Geometry: final body of the model. Coordinates: model frame, mm. Face numbers are marked on the shaded views. A direction names the side the tool comes from. Coordinates: 2 decimals unless noted, no trailing zeros. Write each loop counter-clockwise with the first axis right and the second up, starting at its lowest first coordinate (ties: lowest second). Pieces come first, ordered by that corner, then holes. Notation, with made-up numbers: (19.5, 18.25) - (23.5, 18.25) arc R7 ccw to (23.5, 28.25) - close; hole circle Ø11 at (-20.75, 32). An arc over 180 degrees is marked (long way). Put each result on its own line as item: value.
```python
from build123d import *

# Parameters (mm, degrees)
F0_R     = 11.049
F1_DEPTH = 6.35


with BuildPart() as f1:
    # F0 (on Top) → F1 (new body)
    with BuildSketch(Plane.XY):
        with BuildLine():
            ThreePointArc((13.9900267073, 42.191013886), (7.0856169162, 43.8816195339), (1.001e-07, 44.45))
            ThreePointArc((1.001e-07, 44.45), (-8.1127014874, 43.7033931701), (-15.9528722093, 41.4886534883))
            ThreePointArc((-15.9528722093, 41.4886534883), (-18.8508822531, 32.2986856143), (-16.6280791163, 22.9224860668))
            ThreePointArc((-16.6280791163, 22.9224860668), (-15.8658789133, 20.1464210948), (-15.6090878752, 17.2790975622))
            ThreePointArc((-15.6090878752, 17.2790975622), (-17.5525161747, 9.6016065701), (-22.9146844129, 3.773405023))
            ThreePointArc((-22.9146844129, 3.773405023), (-24.5849396697, 2.8183178083), (-26.356998831, 2.0688176155))
            ThreePointArc((-26.356998831, 2.0688176155), (-36.5044925545, -0.529991355), (-43.6973944973, -8.1449502237))
            ThreePointArc((-43.6973944973, -8.1449502237), (-41.7877364398, -15.1521478094), (-38.7624793768, -21.7548314763))
            ThreePointArc((-38.7624793768, -21.7548314763), (-29.6282610574, -1.7859753114), (-12.3702381212, -15.3635231449))
            ThreePointArc((-12.3702381212, -15.3635231449), (-22.3396426217, -28.7484450965), (-38.018933275, -23.0296159897))
            ThreePointArc((-38.018933275, -23.0296159897), (-32.9149121168, -29.8732499126), (-26.5966764592, -35.6148747201))
            ThreePointArc((-26.5966764592, -35.6148747201), (-18.7298982199, -33.736427955), (-12.3747177422, -28.7337843329))
            ThreePointArc((-12.3747177422, -28.7337843329), (-12.1077253896, -26.8478523844), (-11.5717802867, -25.020070374))
            ThreePointArc((-11.5717802867, -25.020070374), (-1.3693127664, -16.6255914205), (10.9906537522, -21.2934440388))
            ThreePointArc((10.9906537522, -21.2934440388), (12.2133658929, -23.0689970739), (13.13038636, -25.020070374))
            ThreePointArc((13.13038636, -25.020070374), (20.2980282513, -31.3766165327), (29.7323518206, -33.0422419823))
            ThreePointArc((29.7323518206, -33.0422419823), (33.8520296012, -28.8069885944), (37.3735987968, -24.0627640345))
            ThreePointArc((37.3735987968, -24.0627640345), (13.3667253576, -10.5788234649), (40.5015365819, -15.2530769271))
            ThreePointArc((40.5015365819, -15.2530769271), (40.2743565397, -17.7622201291), (39.6002052135, -20.1897559927))
            ThreePointArc((39.6002052135, -20.1897559927), (42.1478196292, -14.1196246586), (43.7709726947, -7.7397964674))
            ThreePointArc((43.7709726947, -7.7397964674), (37.7292227786, -0.852924429), (29.046183452, 2.0688176155))
            ThreePointArc((29.046183452, 2.0688176155), (27.1074059125, 1.9329851963), (25.168628373, 2.0688176155))
            ThreePointArc((25.168628373, 2.0688176155), (15.5450488675, 8.1144987903), (13.6462865444, 19.3197763418))
            ThreePointArc((13.6462865444, 19.3197763418), (14.2680191104, 21.1739149673), (15.1437362656, 22.9224860668))
            ThreePointArc((15.1437362656, 22.9224860668), (17.3461160042, 32.7231575742), (13.9900267073, 42.191013886))
        make_face()
        with BuildLine():
            ThreePointArc((14.0337661536, -0.0455333574), (-9.7919450545, -9.9463341625), (0, 13.9243211114))
            ThreePointArc((0, 13.9243211114), (9.9194773617, 9.8552674478), (14.0337661536, -0.0455333574))
        make_face(mode=Mode.SUBTRACT)
        with BuildLine():
            ThreePointArc((13.97, 30.48), (9.8782817332, 20.6017182668), (0, 16.51))
            ThreePointArc((0, 16.51), (-13.97, 30.4800000501), (1.001e-07, 44.45))
            ThreePointArc((1.001e-07, 44.45), (9.8782817686, 40.3582816978), (13.97, 30.48))
        make_face(mode=Mode.SUBTRACT)
        with BuildLine():
            ThreePointArc((14.0337661536, -0.0455333574), (9.9194773617, 9.8552674478), (0, 13.9243211114))
            ThreePointArc((0, 13.9243211114), (-9.7919450545, -9.9463341625), (14.0337661536, -0.0455333574))
        make_face()
        with BuildLine():
            ThreePointArc((0, 11.049), (7.8128228253, 7.8128228253), (11.049, 0))
            ThreePointArc((11.049, 0), (-7.8128228253, -7.8128228253), (0, 11.049))
        make_face(mode=Mode.SUBTRACT)
        with BuildLine():
            ThreePointArc((1.001e-07, 44.45), (-13.97, 30.4800000501), (0, 16.51))
            ThreePointArc((0, 16.51), (9.8782817332, 20.6017182668), (13.97, 30.48))
            ThreePointArc((13.97, 30.48), (9.8782817686, 40.3582816978), (1.001e-07, 44.45))
        make_face()
        with BuildLine():
            ThreePointArc((11.049, 30.48), (7.8128228253, 22.6671771747), (0, 19.431))
            ThreePointArc((0, 19.431), (-7.8128228253, 38.2928228253), (11.049, 30.48))
        make_face(mode=Mode.SUBTRACT)
        with BuildLine():
            ThreePointArc((-12.3702381212, -15.3635231449), (-29.6282610574, -1.7859753114), (-38.7624793768, -21.7548314763))
            ThreePointArc((-38.7624793768, -21.7548314763), (-38.3959972014, -22.3953097524), (-38.018933275, -23.0296159897))
            ThreePointArc((-38.018933275, -23.0296159897), (-22.3396426217, -28.7484450965), (-12.3702381212, -15.3635231449))
        make_face()
        with Locations((-26.3402381212, -15.3635231449)):
            Circle(F0_R, mode=Mode.SUBTRACT)
        with BuildLine():
            ThreePointArc((37.3735987968, -24.0627640345), (38.5355897032, -22.1542507484), (39.6002052135, -20.1897559927))
            ThreePointArc((39.6002052135, -20.1897559927), (40.2743565397, -17.7622201291), (40.5015365819, -15.2530769271))
            ThreePointArc((40.5015365819, -15.2530769271), (13.3667253576, -10.5788234649), (37.3735987968, -24.0627640345))
        make_face()
        with Locations((26.5315365819, -15.2530769271)):
            Circle(F0_R, mode=Mode.SUBTRACT)
        with BuildLine():
            ThreePointArc((-38.7624793768, -21.7548314763), (-41.7877364398, -15.1521478094), (-43.6973944973, -8.1449502237))
            ThreePointArc((-43.6973944973, -8.1449502237), (-42.9395681626, -26.7309598149), (-26.5966764592, -35.6148747201))
            ThreePointArc((-26.5966764592, -35.6148747201), (-32.9149121168, -29.8732499126), (-38.018933275, -23.0296159897))
            ThreePointArc((-38.018933275, -23.0296159897), (-38.4075515273, -22.4020490671), (-38.7624793768, -21.7548314763))
        make_face()
        with BuildLine():
            ThreePointArc((-11.5717802867, -25.020070374), (-12.1077253896, -26.8478523844), (-12.3747177422, -28.7337843329))
            ThreePointArc((-12.3747177422, -28.7337843329), (1.7565735529, -36.3458547771), (13.13038636, -25.020070374))
            ThreePointArc((13.13038636, -25.020070374), (12.2133658929, -23.0689970739), (10.9906537522, -21.2934440388))
            ThreePointArc((10.9906537522, -21.2934440388), (1.0648132035, -31.3627294368), (-11.5717802867, -25.020070374))
        make_face()
        with BuildLine():
            ThreePointArc((29.046183452, 2.0688176155), (29.875596689, 17.6827436404), (15.1437362656, 22.9224860668))
            ThreePointArc((15.1437362656, 22.9224860668), (14.2680191104, 21.1739149673), (13.6462865444, 19.3197763418))
            ThreePointArc((13.6462865444, 19.3197763418), (26.0608319773, 15.138250311), (25.168628373, 2.0688176155))
            ThreePointArc((25.168628373, 2.0688176155), (27.1074059125, 1.9329851963), (29.046183452, 2.0688176155))
        make_face()
        with BuildLine():
            ThreePointArc((-15.6090878752, 17.2790975622), (-15.8658789133, 20.1464210948), (-16.6280791163, 22.9224860668))
            ThreePointArc((-16.6280791163, 22.9224860668), (-31.7457216544, 17.2790975622), (-26.356998831, 2.0688176155))
            ThreePointArc((-26.356998831, 2.0688176155), (-24.5849396697, 2.8183178083), (-22.9146844129, 3.773405023))
            ThreePointArc((-22.9146844129, 3.773405023), (-28.3246437936, 15.4285434715), (-15.6090878752, 17.2790975622))
        make_face()
        with BuildLine():
            ThreePointArc((-15.9528722093, 41.4886534883), (-8.1127014874, 43.7033931701), (1.001e-07, 44.45))
            ThreePointArc((1.001e-07, 44.45), (7.0856169162, 43.8816195339), (13.9900267073, 42.191013886))
            ThreePointArc((13.9900267073, 42.191013886), (-1.1671052189, 49.7558144069), (-15.9528722093, 41.4886534883))
        make_face()
        with BuildLine():
            ThreePointArc((29.7323518206, -33.0422419823), (43.3672029043, -24.0615366442), (43.7709726947, -7.7397964674))
            ThreePointArc((43.7709726947, -7.7397964674), (42.1478196292, -14.1196246586), (39.6002052135, -20.1897559927))
            ThreePointArc((39.6002052135, -20.1897559927), (38.6427219172, -22.2158414481), (37.3735987968, -24.0627640345))
            ThreePointArc((37.3735987968, -24.0627640345), (33.8520296012, -28.8069885944), (29.7323518206, -33.0422419823))
        make_face()
    extrude(amount=F1_DEPTH)


solid = f1.part
```
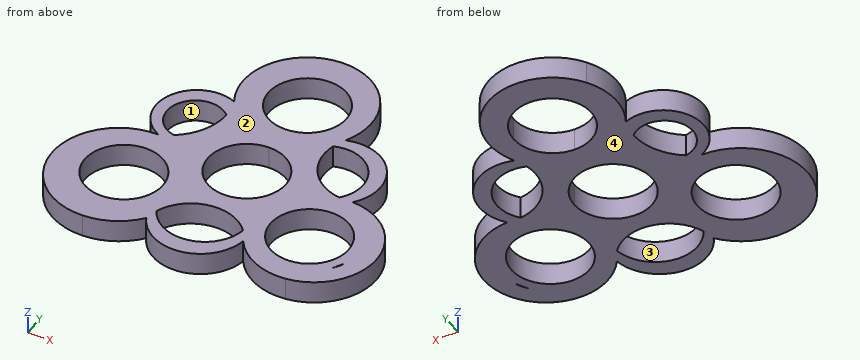
1. Section query A-A (y = 29). Return loops of the section in (x, z), then the cut area to 3 significant figures.
Answer below:
outline: (-18.67, 0) - (-10.95, 0) - (-10.95, 6.35) - (-18.67, 6.35) - close; (10.95, 0) - (17.19, 0) - (17.19, 6.35) - (10.95, 6.35) - close
area: 88.6 mm²
2. Set-up query: the marked faces 3 and 4. Return all of +Z, -Z, +X, -X, +Y, -Y with unobstructed straight access to the full face (end or side cutting, diameter ignored); none if empty.
Answer below:
face 3: +Z, -Z
face 4: -Z, +X, -X, +Y, -Y
3. Ray query, probe 1 along X at (y, z) = (-6, 4.5); probe 2 along X at (y, z) = (6, 2.5); probe 3 along Y at (x, z) = (8, 5.25). Return the intervals inside material, ascending. Write a range as from..to.
Answer below:
probe 1: x = -42.41..-32.21, -20.47..-9.28, 9.28..20.49, 32.57..42.79
probe 2: x = -30.87..-26.99, -20.21..-9.28, 9.28..17.28, 27.38..31.3
probe 3: y = -33.71..-27.59, -18.6..-7.62, 7.62..22.86, 38.1..47.51
4. Section query C-C (z = 4). Count the separate pieces of the cut face and the enclosed holes in it, then the cut area to 3 significant figures.
Answer below:
separate pieces: 1
enclosed holes: 9
area: 2,950 mm²
5. Mould query, pull axis X, two halves, no side actions, for the marked faces 1 and 2. Classes: +X half, -X half, draft (parallel to the pull), parting line (faces both ways), or undercut.
Answer below:
face 1: undercut
face 2: draft
6. Section query B-B (x = 4.5). Return loops of the section in (y, z), then the cut area to 3 significant figures.
Answer below:
outline: (-35.65, 0) - (-30.25, 0) - (-30.25, 6.35) - (-35.65, 6.35) - close; (-16.99, 0) - (-10.09, 0) - (-10.09, 6.35) - (-16.99, 6.35) - close; (10.09, 0) - (20.39, 0) - (20.39, 6.35) - (10.09, 6.35) - close; (40.57, 0) - (48.99, 0) - (48.99, 6.35) - (40.57, 6.35) - close
area: 197 mm²
7. Pin query (flat end, axial travel): pin 1 Ø13.5 at (x, y) = (-26.34, -15.36) entering from -Z. Return the tip coordinate at first contact, or that it passes through.
Answer below:
pin 1: passes through
8. Section query D-D (y = 13). Return loops of the section in (x, z), then the cut area to 3 significant figures.
Answer below:
outline: (-32.81, 0) - (-29.17, 0) - (-29.17, 6.35) - (-32.81, 6.35) - close; (-16.19, 0) - (13.5, 0) - (13.5, 6.35) - (-16.19, 6.35) - close; (27.16, 0) - (31.82, 0) - (31.82, 6.35) - (27.16, 6.35) - close
area: 241 mm²
